from build123d import *

# Parameters (mm, degrees)
BOSS_EXTRU_1_DEPTH             = 10
CBORE_FOR_M2_SHCS1_D           = 2.5
CBORE_FOR_M2_SHCS1_CBORE_D     = 4.25
CBORE_FOR_M2_SHCS1_CBORE_DEPTH = 8.5
CONG_1_R                       = 0.5
ESQUISSE6_R                    = 1.6
ENL_V_MAT_EXTRU_1_DEPTH        = 19.791620526
ESQUISSE7_W                    = 5.85
ESQUISSE7_H                    = 2.25
ENL_V_MAT_EXTRU_2_DEPTH        = 7.25
SKETCH1_R                      = 4.5
CUT_EXTRUDE1_DEPTH             = 3


with BuildPart() as part:
    # Esquisse1 → Boss.-Extru.1 (new body)
    with BuildSketch(Plane(origin=(0, 0, 0), x_dir=(1, 0, 0), z_dir=(0, 1, 0))):
        with BuildLine():
            Line((6.025985397, 9.5), (-6.025985397, 9.5))
            ThreePointArc((-6.025985397, 9.5), (0, -11.25), (6.025985397, 9.5))
        make_face()
        with BuildLine():
            Line((-3.225, 0), (-3.225, 2.9))
            Line((-3.225, 2.9), (3.225, 2.9))
            Line((3.225, 2.9), (3.225, 0))
            ThreePointArc((3.225, 0), (0, -3.225), (-3.225, 0))
        make_face(mode=Mode.SUBTRACT)
    extrude(amount=BOSS_EXTRU_1_DEPTH)

    # CBORE for M2 SHCS1 (through all)
    with Locations(Plane(origin=(0, 10, 0), x_dir=(1, 0, 0), z_dir=(0, 1, 0))):
        with Locations((8, 0), (-8, 0), (0, 0), (0, -8)):
            CounterBoreHole(CBORE_FOR_M2_SHCS1_D / 2, CBORE_FOR_M2_SHCS1_CBORE_D / 2, CBORE_FOR_M2_SHCS1_CBORE_DEPTH)

    # Congé1
    cong_1_edges = [part.edges().sort_by_distance(p)[0] for p in [
        (0, 10, 3.225),
        (3.225, 10, -1.45),
        (0, 10, -2.9),
        (-3.225, 10, -1.45),
    ]]
    fillet(cong_1_edges, radius=CONG_1_R)

    # Esquisse6 → Enlèv. mat.-Extru.1 (cut, through all)
    with BuildSketch(Plane.XY):
        with Locations((0, 4.5)):
            Circle(ESQUISSE6_R)
    extrude(amount=-ENL_V_MAT_EXTRU_1_DEPTH, mode=Mode.SUBTRACT)

    # Esquisse7 → Enlèv. mat.-Extru.2 (cut)
    with BuildSketch(Plane(origin=(0, 0, 0), x_dir=(1, 0, 0), z_dir=(0, 1, 0))):
        with Locations((0, 5.525)):
            Rectangle(ESQUISSE7_W, ESQUISSE7_H)
    extrude(amount=ENL_V_MAT_EXTRU_2_DEPTH, mode=Mode.SUBTRACT)

    # Sketch1 → Cut-Extrude1 (cut)
    with BuildSketch(Plane.XZ):
        Circle(SKETCH1_R)
    extrude(amount=-CUT_EXTRUDE1_DEPTH, mode=Mode.SUBTRACT)


solid = part.part
Can you work these out from the model? Positions are in its coordinate system, mm. A direction names the side the tool comes from. Coordinates: 2 decimals unless noted, no trailing zeros. Order: outer loops, then holes, each group sorted by start corner. A loop starts at its lowest first (then second) coordinate and runs counter-clockwise, first axis right, second up. Notation, with made-up numbers: M 26.5,9.5 L 82.5,9.5 A14 cw 82.5,25.5 Z; hole C 12,74 d1. An arc over 180 degrees is marked long. Write item = value, one per line.
(1) If we mould it in two halves opening along X, with no side actions, what happens to faces 6 (the face through (-3, 10, 3)), 7 (the face through (9.142, 5.81, -1.792))? For each: pulls with the +X half, pulls with the -X half, needs draft (parallel to the pull), parting line crosses it, or undercut.
Results are:
face_6 = needs draft
face_7 = undercut
(2) Suppose I cut it at C-C on z = 8. Please give me the cut outline in (x, y) (3 decimals), plus the area to 3 significant figures.
Results are:
outline = M -7.91,0 L -1.25,0 L -1.25,1.5 L -2.125,1.5 L -2.125,10 L -7.91,10 Z; M 1.25,0 L 7.91,0 L 7.91,10 L 2.125,10 L 2.125,1.5 L 1.25,1.5 Z
area = 118 mm2
(3) For faces 1 (the face through (-7, 1.5, 1)), 2 (the face through (0.06, 6.1, -3.64)), 3 (the face through (0.185, 1.479, 4.496)), 4 (the face through (-3.225, 6, -1)), 5 (the face through (0, 0, 5)), which set-ups out of +Z, -Z, +X, -X, +Y, -Y let a thin tool reach every point of the face, with its end or its side?
Results are:
face_1 = +Y
face_2 = -Z
face_3 = -Y
face_4 = +Y, -Y
face_5 = +Z, -Z, +X, -X, -Y
(4) For pin 1 Ø2 at (x, z) = (8.5, 0.5) entering from +Y; pin 2 Ø2.5 at (y, z) = (5.5, -1.5) entering from -X; pin 3 Ø2 at (x, y) = (-2, 8) entering from +Z, each with a flat end and sliding along its axis, tell me the tip position at first contact or that it passes through.
Results are:
pin_1 = 1.5
pin_2 = -11.25
pin_3 = 11.21
(5) Suppose I cut it at B-B on y = 4.5. Please give me the cut outline in (x, z) (3 decimals).
Results are:
outline = M -6.026,-9.5 L -1.6,-9.5 L -1.6,-6.65 L -2.925,-6.65 L -2.925,-4.4 L -1.6,-4.4 L -1.6,-2.9 L -3.225,-2.9 L -3.225,0 A3.225 cw 3.225,0 L 3.225,-2.9 L 1.6,-2.9 L 1.6,-4.4 L 2.925,-4.4 L 2.925,-6.65 L 1.6,-6.65 L 1.6,-9.5 L 6.026,-9.5 A11.25 ccw long Z; hole C -8,0 d4.25; hole C 0,8 d4.25; hole C 8,0 d4.25
(6) I need wall thicknesses on line 1 along Z through (x, y) = (-1.75, 8); line 2 along Z through (x, y) = (-8, 5) (3 decimals); line 3 along Y through (x, z) = (-7.5, 1.75). Which ranges of each line are inside material? Lowest first, please. Write a range as [from, to].
Results are:
line_1 = [-9.5, -2.9], [2.71, 6.79], [9.21, 11.11]
line_2 = [-7.91, -2.125], [2.125, 7.91]
line_3 = [0, 1.5]
(7) Suppose I cut it at D-D on x = -8. Please give me the cut outline in (y, z) (3 decimals).
Results are:
outline = M 0,-7.91 L 10,-7.91 L 10,-2.125 L 1.5,-2.125 L 1.5,-1.25 L 0,-1.25 Z; M 0,1.25 L 1.5,1.25 L 1.5,2.125 L 10,2.125 L 10,7.91 L 0,7.91 Z
(8) Suppose I cut it at A-A on y = 8.25. Please give me the cut outline in (x, z) (3 decimals), plus the area to 3 significant figures.
Results are:
outline = M -6.026,-9.5 L 6.026,-9.5 A11.25 ccw long Z; hole C -8,0 d4.25; hole M -3.225,-2.9 L 3.225,-2.9 L 3.225,0 A3.225 ccw -3.225,0 Z; hole C 0,8 d4.25; hole C 8,0 d4.25
area = 306 mm2
